Input: part model. Units: mm. Frame: model coordinates. A direction names the side the tool comes from. Coordinates: 2 decimals unless noted, no trailing zeros. Loops run counter-clockwise (first coordinate to the right, second up) from the corner with the lowest first, then second, coordinate; pieces in that order, holes last.
(1) Line query: L1, parallel to Y at x = -33, z = -24.5; L2, parallel to Y at x = -20, z = -5.5; L3, parallel to X at y = 25.5, z = -19. Output: solid intervals per line, ascending.
(2) Set-up query: faces 4 (the face through (46.859, 35.181, -20.036)), 5 (the face through (56.747, 24, 0)), 6 (the face through (36.747, 24, 0)), 7 (the face through (-18, 20, -23)). Return all of +Z, -Z, +X, -X, +Y, -Y with unobstructed straight access to the full face (end or side cutting, diameter ignored); none if empty.
(3) Mould query, pull axis X, two halves, no side actions, for faces 1 (the face through (-1, 10, 50)), 2 (the face through (38.747, 31, -8)), 3 (the face through (54.747, 31, -8)). Classes: released by +X, released by -X, zero draft, split by the parting line, or undercut.
(4) Section A-A, the plane x = 0. Return loops of the section in (y, z), then the cut area to 3 significant figures.
(5) Section B-B, the plane z = -10. Return loops of the section in (x, y), then the cut area to 3 significant figures.
(6) Section C-C, the plane y = 35.5. Return loops of the section in (x, z), then the cut area to 3 significant figures.
(7) Section D-D, the plane y = 49. Return loops of the section in (x, z), then the cut area to 3 significant figures.
(8) Contact query for flat-ended pins moving along their axis: P1, Ø8, axis at y = 22, z = -3, coming from the -X side; P2, Ø6.5, axis at y = 33, z = 7.5, coming from the +X side; P3, Ø6, axis at x = 44, y = 23.5, coming from the -Z side; P4, Ø2, axis at y = 25, z = 10.5, coming from the +X side. Output: stop coordinate, or through.
```python
from build123d import *

# Parameters (mm, degrees)
SKETCH1_W            = 150
SKETCH1_H            = 100
BOSS_EXTRUDE1_DEPTH  = 20
SKETCH2_R            = 24.239154651
BOSS_EXTRUDE2_DEPTH  = 40
SKETCH3_R            = 5.073901121
BOSS_EXTRUDE3_DEPTH  = 100
SKETCH17_W           = 20
SKETCH17_H           = 48.5
BOSS_EXTRUDE14_DEPTH = 7.5
BOSS_EXTRUDE15_START = -2
BOSS_EXTRUDE15_DEPTH = 16
FILLET5_START        = 38.747344483
FILLET5_DEPTH        = 16


with BuildPart() as part:
    # Sketch1 → Boss-Extrude1 (new body)
    with BuildSketch(Plane(origin=(0, 0, 0), x_dir=(1, 0, 0), z_dir=(0, 1, 0))):
        Rectangle(SKETCH1_W, SKETCH1_H)
    extrude(amount=BOSS_EXTRUDE1_DEPTH)

    # Sketch2 → Boss-Extrude2 (add)
    with BuildSketch(Plane(origin=(0, 0, 0), x_dir=(1, 0, 0), z_dir=(0, 1, 0))):
        with Locations(Location((0, 0, 0), (0, 0, 270))):
            Circle(SKETCH2_R)
    extrude(amount=BOSS_EXTRUDE2_DEPTH)

    # Sketch3 → Boss-Extrude3 (add)
    with BuildSketch(Plane(origin=(0, 0, 0), x_dir=(1, 0, 0), z_dir=(0, 1, 0))):
        with Locations(Location((0, 0, 0), (0, 0, 90))):
            Circle(SKETCH3_R)
    extrude(amount=BOSS_EXTRUDE3_DEPTH)

    # Sketch5 → Revolve2 (revolve)
    with BuildSketch(Plane(origin=(0, 0, 0), x_dir=(0, 0, -1), z_dir=(1, 0, 0))):
        with BuildLine():
            Line((0.229753848, 98.790742156), (0.229753848, 128.790742156))
            ThreePointArc((0.229753848, 128.790742156), (-14.770246152, 113.790742156), (0.229753848, 98.790742156))
        make_face()
    revolve(axis=Axis((0, 98.790742156, -0.229753848), (0, 1, 0)))

    # Sketch17 → Boss-Extrude14 (add)
    with BuildSketch(Plane(origin=(0, 20, 0), x_dir=(1, 0, 0), z_dir=(0, 1, 0))):
        with Locations((46.747344483, 0.04322355)):
            Rectangle(SKETCH17_W, SKETCH17_H)
    extrude(amount=BOSS_EXTRUDE14_DEPTH)

    # Sketch21 → Boss-Extrude15 (add)
    with BuildSketch(Plane(origin=(56.747344483, 0, 0), x_dir=(0, 0, -1), z_dir=(1, 0, 0)).offset(BOSS_EXTRUDE15_START)):
        with BuildLine():
            Line((19.134328626, 27.5), (-23.063699683, 27.5))
            ThreePointArc((-23.063699683, 27.5), (-2.634761018, 31.291523365), (16.230010888, 40))
            ThreePointArc((16.230010888, 40), (20.271004522, 34.351503898), (19.134328626, 27.5))
        make_face()
    extrude(amount=-BOSS_EXTRUDE15_DEPTH)

    # Fillet5: read off the stored shape, not the designer's step
    # Fillet5 outline → Fillet5 (add)
    with BuildSketch(Plane.YZ.offset(FILLET5_START)):
        with BuildLine():
            Line((27.5, -19.134328626), (27.5, -20.763165982))
            add(Edge.make_bspline(
                [(27.5, -20.763165982), (27.5, -20.531845888), (27.5, -20.300525794), (27.623544112, -19.810870378), (27.937534857, -19.585621938), (28.467988806, -19.663458549), (28.675738966, -19.755036772), (28.876983932, -19.836946184)],
                knots=[0, 0, 0, 0, 0, 0, 0.5, 0.5, 1, 1, 1, 1, 1, 1], degree=5))
            ThreePointArc((28.876983932, -19.836946184), (28.173502588, -19.515013461), (27.5, -19.134328626))
        make_face()
    extrude(amount=FILLET5_DEPTH)

    # Sketch24 → Revolve3 (revolve)
    with BuildSketch(Plane(origin=(0, 20, 0), x_dir=(1, 0, 0), z_dir=(0, 1, 0))):
        with BuildLine():
            Line((-62.255471135, 39.768833527), (-57.287341541, 39.768833527))
            ThreePointArc((-57.287341541, 39.768833527), (-59.771406338, 42.252898324), (-62.255471135, 39.768833527))
        make_face()
    revolve(axis=Axis((-62.255471135, 20, -39.768833527), (1, 0, 0)))

    # Sketch25 → Revolve4 (revolve)
    with BuildSketch(Plane(origin=(0, 20, 0), x_dir=(1, 0, 0), z_dir=(0, 1, 0))):
        with BuildLine():
            Line((-62.255471135, 29.059615512), (-57.287341541, 29.059615512))
            ThreePointArc((-57.287341541, 29.059615512), (-59.771406338, 31.543680309), (-62.255471135, 29.059615512))
        make_face()
    revolve(axis=Axis((-62.255471135, 20, -29.059615512), (1, 0, 0)))


solid = part.part
```
Report:
1. L1: y = 0 to 20
1. L2: y = 0 to 40
1. L3: x = -15.05 to 15.05, 36.75 to 56.75
2. face 4: -Z, +X
2. face 5: +Z, -Z, +X, +Y
2. face 6: +Z, -Z, +Y
2. face 7: +Y
3. face 1: zero draft
3. face 2: undercut
3. face 3: released by +X
4. outline: (0, -50) - (20, -50) - (20, -24.24) - (40, -24.24) - (40, -5.07) - (99.59, -5.07) arc R15 ccw (long way) to (99.76, 5.07) - (40, 5.07) - (40, 24.24) - (20, 24.24) - (20, 50) - (0, 50) - close
4. area: 4,280 mm2
5. outline: (-75, 0) - (75, 0) - (75, 20) - (56.75, 20) - (56.75, 27.5) - (54.75, 27.5) - (54.75, 36.48) - (38.75, 36.48) - (38.75, 27.5) - (36.75, 27.5) - (36.75, 20) - (22.08, 20) - (22.08, 40) - (-22.08, 40) - (-22.08, 20) - (-75, 20) - close; circle Ø22.76 at (0, 113.79)
5. area: 4,580 mm2
6. outline: circle Ø48.48 at (0, 0); (38.75, -19.92) - (54.75, -19.92) - (54.75, -8.01) - (38.75, -8.01) - close
6. area: 2,040 mm2
7. outline: circle Ø10.15 at (0, 0)
7. area: 80.9 mm2
8. P1: stops at x = -75
8. P2: stops at x = 54.75
8. P3: stops at z = -24.29
8. P4: stops at x = 56.75
